Geometry check sheet. Reference: the model listing, model coordinates, mm. A direction names the side the tool comes from. Coordinates: 2 decimals unless noted, no trailing zeros. Loops run counter-clockwise (first coordinate to the right, second up) from the corner with the lowest first, then second, coordinate; pieces in that order, holes last.
from build123d import *

# Parameters (mm, degrees)
BOSS_EXTRUDE1_DEPTH              = 25
FILLET1_R                        = 25
SKETCH4_W                        = 61.258938573
SKETCH4_H                        = 20
CUT_EXTRUDE1_DEPTH               = 50
SKETCH5_W                        = 61.074850192
SKETCH5_H                        = 20
CUT_EXTRUDE2_DEPTH               = 50
F_20_0MM_DOWEL_HOLE1_D           = 20
F_20_0MM_DOWEL_HOLE1_ON_FACE_2_D = 20


with BuildPart() as part:
    # Sketch1 → Boss-Extrude1 (new, symmetric)
    with BuildSketch(Plane.XY):
        with BuildLine():
            Line((-150, 25), (0, 25))
            Line((0, 25), (0, -25))
            Line((0, -25), (-149.999982985, -25))
            ThreePointArc((-149.999982985, -25), (-174.999982985, -8.507e-06), (-150, 25))
        make_face()
    extrude(amount=BOSS_EXTRUDE1_DEPTH, both=True)

    # Fillet1
    fillet1_edges = [part.edges().sort_by_distance(p)[0] for p in [
        (0, 0, -25),
        (0, 0, 25),
    ]]
    fillet(fillet1_edges, radius=FILLET1_R - 0.0001)  # a hair under: the kernel refuses the full size

    # Sketch4 → Cut-Extrude1 (cut)
    with BuildSketch(Plane(origin=(0, 25, 0), x_dir=(1, 0, 0), z_dir=(0, 1, 0))):
        with Locations((-155.629452272, 0)):
            Rectangle(SKETCH4_W, SKETCH4_H)
    extrude(amount=-CUT_EXTRUDE1_DEPTH, mode=Mode.SUBTRACT)

    # Sketch5 → Cut-Extrude2 (cut)
    with BuildSketch(Plane(origin=(0, 0, -25), x_dir=(-1, 0, 0), z_dir=(0, 0, -1))):
        with Locations((19.462574904, 0)):
            Rectangle(SKETCH5_W, SKETCH5_H)
    extrude(amount=-CUT_EXTRUDE2_DEPTH, mode=Mode.SUBTRACT)

    # Ø20.0mm Dowel Hole1 (through all)
    with Locations(Plane(origin=(-149.999982985, 0, 25), x_dir=(1, 0, 0), z_dir=(0, 0, 1))):
        with Locations((0, 0)):
            Hole(F_20_0MM_DOWEL_HOLE1_D / 2)

    # Ø20.0mm Dowel Hole1 on face 2 (through all)
    with Locations(Plane(origin=(-25, -25, 0), x_dir=(0, 0, -1), z_dir=(0, -1, 0))):
        with Locations((0, 0)):
            Hole(F_20_0MM_DOWEL_HOLE1_ON_FACE_2_D / 2)


solid = part.part
1) Section check B-B on y = 0. Record the cut outline in (x, z).
Data:
outline: (-175, -25) - (-160, -25) - (-160, -10) - (-175, -10) - close; (-175, 10) - (-160, 10) - (-160, 25) - (-175, 25) - close; (-140, -25) - (-50, -25) - (-50, 25) - (-140, 25) - (-140, 10) - (-125, 10) - (-125, -10) - (-140, -10) - close
2) Access from +Z, -Z, +X, -X, +Y, -Y to the whole of each face (thin tool, end or side, straight path). Record for faces 5 (the flat face through (-99, 0, 25)), 6 (the flat face through (-139, 0, -10)), 7 (the flat face through (-36, 10, 0)).
Data:
face 5: +Z, +X, -X, +Y, -Y
face 6: -X, +Y, -Y
face 7: +Z, -Z, +X
3) Section check C-C on x = -22.5. Record the cut outline in (y, z), and give its area (3 significant figures).
Data:
outline: (-25, -24.87) - (-10, -24.87) - (-10, -9.68) - (-25, -9.68) - close; (-25, 9.68) - (-10, 9.68) - (-10, 24.87) - (-25, 24.87) - close; (10, -24.87) - (25, -24.87) - (25, -9.68) - (10, -9.68) - close; (10, 9.68) - (25, 9.68) - (25, 24.87) - (10, 24.87) - close
area: 912 mm2
4) Depth check by flat-ended pin: pin 1 (8 mm diameter, centred on y = -2, z = -9.5, fed in from -X); pin 2 (10 mm diameter, centred on y = 2.5, z = -4, fed in from -X); pin 3 (10 mm diameter, centred on y = -1, z = 3, fed in from +X). Enter the tip coordinate at first touch or a pass-through.
Data:
pin 1: stops at x = -175
pin 2: stops at x = -125
pin 3: stops at x = -50
5) Mould release check, pull along X, two halves, no side actions. Record for faces 1 (the cylindrical face through (-7.129, 17.395, -17.482)), 2 (the flat face through (-36, -10, 0)), 3 (the cylindrical face through (-159.237, -3.83, 17.395)), 4 (the flat face through (-125, 0, 0)): +X half, -X half, draft (parallel to the pull), parting line (faces both ways), or undercut.
Data:
face 1: +X half
face 2: draft
face 3: undercut
face 4: -X half
6) Section check A-A on x = -40. Record the cut outline in (y, z).
Data:
outline: (-25, -25) - (-10, -25) - (-10, 25) - (-25, 25) - close; (10, -25) - (25, -25) - (25, 25) - (10, 25) - close
7) Section check D-D on z = -14. Record the cut outline in (x, y), and give its area (3 significant figures).
Data:
outline: (-150, -25) - (-4.29, -25) - (-4.29, -10) - (-50, -10) - (-50, 10) - (-4.29, 10) - (-4.29, 25) - (-150, 25) arc R25 ccw to start; hole circle Ø20 at (-150, 0)
area: 7,040 mm2
8) Material ranges on probe 1 along X at (y, z) = (21, 0); probe 2 along Z at (x, y) = (-127, 1.5), recorded low to high.
Data:
probe 1: x = -125 to -35, -15 to 0
probe 2: z = -25 to -10, 10 to 25
